Here's how the part is built. I have some questions about the finished solid (model axes, mm). Coordinates: 2 decimals unless noted, no trailing zeros. Loops run counter-clockwise (first coordinate to the right, second up) from the corner with the lowest first, then second, coordinate; pieces in that order, holes last. Notation, with made-up numbers: M 34,79 L 48,79 A15 cw 48,101 Z; hole C -14,43.25 d10. An arc over 180 degrees is marked long. Use one line per item in the form item = value. Start each with the question number.
(1) Imagine slicing it at A-A, the plane y = 0. Please give me the cut outline in (x, z), and give its area (3 significant figures).
(2) Imagine slicing it at D-D, the plane z = -69. Please give me the cut outline in (x, y).
(3) Will these pins go through, and if not, where does the flat tip stop? P1, Ø1, axis at x = 2.5, z = -189, coming from the +Y side; P2, Ø17.5, axis at y = 0, z = -265, coming from the +X side; P3, Ø3, axis at x = 4, y = -13.5, coming from the -Z side.
(4) Imagine slicing it at B-B, the plane z = -125.5. Please give me the cut outline in (x, y).
(5) Thinking about a two-plate mould opening in Z: for faces 1 (the cylindrical face through (3.13, 0.48, -121.51)), 2 (the cylindrical face through (3, 0, 16)), 3 (the flat face through (3.131, 20.056, -197.822)), which applies, +Z half, -Z half, draft (parallel to the pull), parting line (faces both ways), or undercut?
(6) Imagine slicing it at C-C, the plane x = 5. Please give me the cut outline in (y, z).
(7) Please list where these lines run through material, in increasing order: L1, parallel to Y at x = 2.5, z = -132.5; L2, parallel to Z at x = 4.75, y = 3; L3, parallel to Y at x = 2, z = -265.
```python
from build123d import *

# Parameters (mm, degrees)
SKETCH1_R           = 11
BOSS_EXTRUDE1_DEPTH = 6.35


with BuildPart() as part:
    # Sketch1 → Boss-Extrude1 (new body)
    with BuildSketch(Plane(origin=(0, 0, 0), x_dir=(0, 0, -1), z_dir=(1, 0, 0))):
        with BuildLine():
            Line((0, 16), (132.5, 24))
            Line((132.5, 24), (265, 16))
            ThreePointArc((265, 16), (281, 0), (265, -16))
            Line((265, -16), (132.5, -24))
            Line((132.5, -24), (0, -16))
            ThreePointArc((0, -16), (-16, 0), (0, 16))
        make_face()
        Circle(SKETCH1_R, mode=Mode.SUBTRACT)
        with Locations((265, 0)):
            Circle(SKETCH1_R, mode=Mode.SUBTRACT)
        with Locations((132.5, 0)):
            Circle(SKETCH1_R, mode=Mode.SUBTRACT)
    extrude(amount=BOSS_EXTRUDE1_DEPTH)


solid = part.part
```
Answer:
q1.outline = M 0,-281 L 6.35,-281 L 6.35,-276 L 0,-276 Z; M 0,-254 L 6.35,-254 L 6.35,-143.5 L 0,-143.5 Z; M 0,-121.5 L 6.35,-121.5 L 6.35,-11 L 0,-11 Z; M 0,11 L 6.35,11 L 6.35,16 L 0,16 Z
q1.area = 1,470 mm²
q2.outline = M 0,-20.17 L 6.35,-20.17 L 6.35,20.17 L 0,20.17 Z
q3.P1 = 20.62
q3.P2 = through
q3.P3 = -275.58
q4.outline = M 0,-23.58 L 6.35,-23.58 L 6.35,-8.49 L 0,-8.49 Z; M 0,8.49 L 6.35,8.49 L 6.35,23.58 L 0,23.58 Z
q5.face_1 = undercut
q5.face_2 = +Z half
q5.face_3 = -Z half
q6.outline = M -24,-132.5 L -16,-265 A16 ccw 16,-265 L 24,-132.5 L 16,0 A16 ccw -16,0 Z; hole C 0,-265 d22; hole C 0,-132.5 d22; hole C 0,0 d22
q7.L1 = -24 to -11, 11 to 24
q7.L2 = -280.72 to -275.58, -254.42 to -143.08, -121.92 to -10.58, 10.58 to 15.72
q7.L3 = -16 to -11, 11 to 16
